For this review, take the finished solid that the model builds, in its own axes (mm). Round coordinates to 2 decimals unless told otherwise and drop trailing zeros. Order: outer loops, then holes, each group sorted by start corner. A loop starts at its lowest first (then second) coordinate and runs counter-clockwise, first axis right, second up.
Autodesk Inventor part; units mm, degrees
ref_plane "YZ Plane" through (0, 0, 0) normal (1, 0, 0) x (0, 1, 0)
ref_plane "XZ Plane" through (0, 0, 0) normal (0, 1, 0) x (-1, 0, 0)
ref_plane "XY Plane" through (0, 0, 0) normal (0, 0, 1) x (1, 0, 0)
sketch "Эскиз1" plane through (0, 0, 0) normal (0, 1, 0) x (-1, 0, 0)
  line L0 (-25, -140.25) -> (25, -140.25)
  line L1 (25, -140.25) -> (25, 140.25)
  line L2 (25, 140.25) -> (-25, 140.25)
  line L3 (-25, 140.25) -> (-25, -140.25)
  line L4 (-25, -140.25) -> (25, 140.25) construction
  line L5 (25, -140.25) -> (-25, 140.25) construction
  circle A0 centre (19.4, 132.25) radius 1.65
  circle A1 centre (19.4, 92.25) radius 1.65
  line L6 (-25, 0) -> (0, 0)
  line L7 (25, 87.25) -> (19.4, 87.25)
  line L8 (19.4, 87.25) -> (19.4, 67.25)
  line L9 (19.4, 67.25) -> (25, 67.25)
  line L10 (25, 67.25) -> (25, 87.25)
  line L11 (-9.2, 133.25) -> (-2.2, 133.25)
  line L12 (-2.2, 133.25) -> (-2.2, 87.25)
  line L13 (-2.2, 87.25) -> (-9.2, 87.25)
  line L14 (-9.2, 87.25) -> (-9.2, 133.25)
  circle A2 centre (19.4, -132.25) radius 1.65
  circle A3 centre (19.4, -92.25) radius 1.65
  line L15 (25, -87.25) -> (19.4, -87.25)
  line L16 (19.4, -87.25) -> (19.4, -67.25)
  line L17 (19.4, -67.25) -> (25, -67.25)
  line L18 (-9.2, -133.25) -> (-2.2, -133.25)
  line L19 (-2.2, -133.25) -> (-2.2, -87.25)
  line L20 (-2.2, -87.25) -> (-9.2, -87.25)
  line L21 (-9.2, -87.25) -> (-9.2, -133.25)
  point P0 (25, -87.25)
  point P1 (25, -67.25)
  dimension "d0" = 50
  dimension "d1" = 280.5
  dimension "d2" = 3.3
  dimension "d3" = 3.3
  dimension "d4" = 5.6
  dimension "d5" = 5.6
  dimension "d6" = 8
  dimension "d7" = 40
  dimension "d8" = 20
  dimension "d9" = 5
  dimension "d10" = 5.6
  dimension "d11" = 7
  dimension "d12" = 46
  dimension "d13" = 7
  dimension "d17" = 28.6
extrude "Выдавливание1" add sketch "Эскиз1" along normal blind 4 contours L3 L2 L1 L7 L8 L9 L17 L16 L15 L0
chamfer "Фаска1" distance 2 angle 45 2 edges at (25, 2, -140.25) (25, 2, 140.25)
chamfer "Фаска2" distance 0.5 angle 45 8 edges at (9.2, 2, 87.25) (2.2, 2, 87.25) (9.2, 2, 133.25) (2.2, 2, 133.25) (2.2, 2, -87.25) (2.2, 2, -133.25) (9.2, 2, -133.25) (9.2, 2, -87.25)
chamfer "Фаска3" distance 1 angle 45 4 edges at (-25, 2, -87.25) (-25, 2, -67.25) (-25, 2, 87.25) (-25, 2, 67.25)
sketch "Эскиз2" plane through (0, 0, 0) normal (0, -1, 0) x (1, 0, 0)
  line L0 (-25, -66.25) -> (-25, 66.25)
  line L1 (-25, -66.25) -> (-34.9, -66.25)
  line L2 (-34.9, -66.25) -> (-34.9, 66.25)
  line L3 (-34.9, 66.25) -> (-25, 66.25)
  line L4 (-25, 66.25) -> (-25, -66.25)
  point P0 (0, 0)
  dimension "d27" = 9.9
extrude "Выдавливание2" add sketch "Эскиз2" against normal blind 4
sketch "Эскиз3" plane through (0, 4, 0) normal (0, 1, 0) x (1, 0, 0)
  line L0 (-34.9, -66.25) -> (-34.9, 66.25)
  line L1 (-34.9, -60.25) -> (-30.9, -60.25)
  line L2 (-30.9, -60.25) -> (-30.9, -48.25)
  line L3 (-30.9, -48.25) -> (-34.9, -48.25)
  line L4 (-34.9, -48.25) -> (-34.9, -60.25)
  line L5 (-34.9, -66.25) -> (-25, -66.25)
  line L6 (-34.9, -42.25) -> (-30.9, -42.25)
  line L7 (-30.9, -42.25) -> (-30.9, -30.25)
  line L8 (-30.9, -30.25) -> (-34.9, -30.25)
  line L9 (-34.9, -30.25) -> (-34.9, -42.25)
  line L10 (-34.9, -24.25) -> (-30.9, -24.25)
  line L11 (-30.9, -24.25) -> (-30.9, -12.25)
  line L12 (-30.9, -12.25) -> (-34.9, -12.25)
  line L13 (-34.9, -12.25) -> (-34.9, -24.25)
  line L14 (-34.9, -6.25) -> (-30.9, -6.25)
  line L15 (-30.9, -6.25) -> (-30.9, 5.75)
  line L16 (-30.9, 5.75) -> (-34.9, 5.75)
  line L17 (-34.9, 5.75) -> (-34.9, -6.25)
  line L18 (-34.9, 11.75) -> (-30.9, 11.75)
  line L19 (-30.9, 11.75) -> (-30.9, 23.75)
  line L20 (-30.9, 23.75) -> (-34.9, 23.75)
  line L21 (-34.9, 23.75) -> (-34.9, 11.75)
  line L22 (-34.9, 29.75) -> (-30.9, 29.75)
  line L23 (-30.9, 29.75) -> (-30.9, 41.75)
  line L24 (-30.9, 41.75) -> (-34.9, 41.75)
  line L25 (-34.9, 41.75) -> (-34.9, 29.75)
  line L26 (-34.9, 47.75) -> (-30.9, 47.75)
  line L27 (-30.9, 47.75) -> (-30.9, 59.75)
  line L28 (-30.9, 59.75) -> (-34.9, 59.75)
  line L29 (-34.9, 59.75) -> (-34.9, 47.75)
  point P0 (0, 0)
  point P1 (-32.9, -60.25)
  point P2 (-32.9, -42.25)
  point P3 (-32.9, -24.25)
  point P4 (-32.9, -6.25)
  point P5 (-32.9, 11.75)
  point P6 (-32.9, 29.75)
  point P7 (-32.9, 47.75)
  dimension "d32" = 4
  dimension "d33" = 12
  dimension "d34" = 6
  dimension "d37" = 18
extrude "Выдавливание3" cut sketch "Эскиз3" against normal blind 4
sketch "Эскиз4" plane through (0, 4, 0) normal (0, 1, 0) x (1, 0, 0)
  circle A0 centre (-4.9309, -102.75) radius 1.6
  circle A1 centre (15.0691, -102.75) radius 1.6
  circle A2 centre (-5.0691, 102.75) radius 1.6
  circle A3 centre (14.9309, 102.75) radius 1.6
  point P0 (0, 0)
extrude "Выдавливание4" cut sketch "Эскиз4" against normal blind 10
sketch "Эскиз5" plane through (0, 4, 0) normal (0, 1, 0) x (1, 0, 0)
  circle A0 centre (21, -58.5) radius 1.6
  circle A1 centre (-11, -58.5) radius 1.6
  circle A2 centre (21, 58.5) radius 1.6
  circle A3 centre (-11, 58.5) radius 1.6
  point P0 (0, 0)
extrude "Выдавливание5" cut sketch "Эскиз5" against normal blind 10
properties part number "фанера_жлектроника_новая"
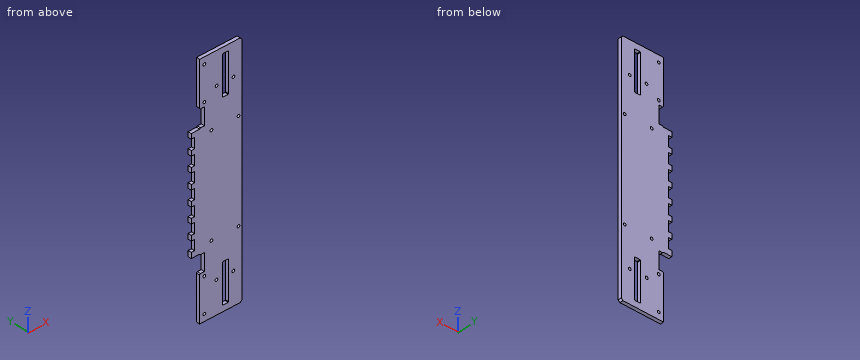
Q1. Take a section at D-D, the plane x = -27.5. State the section outline as (y, z) points.
Q2. Take a section at B-B, the plane z = 83. State the section outline as (x, y) points.
Q3. Take a section at C-C, the plane y = 0.75. Count the separate pieces of the cut face and the enclosed holes in it, plus the area to 3 significant figures.
Q4. Take a section at A-A, the plane z = 123. State the section outline as (x, y) points, plus the area to 3 significant figures.
Q5. Clearance check with flat-ended pins moving along their axes: pin 1 (2 mm diameter, centred on x = -32, y = 2.5, fed in from -Z); pin 2 (2 mm diameter, centred on y = 2.5, z = 51.5, fed in from -X); pin 3 (1.2 mm diameter, centred on y = 2, z = -102, fed in from -X). State where each tip first meets the part, or that it passes through.
Q6. Wall thickness on line 1 (Z direction, x = 21, y = 1.8); line 2 (X direction, y = 1.5, z = 102.75); line 3 (X direction, y = 1.1, z = -132.25): over which ranges is each line inside the solid? List them lowest first.
Working result:
1. outline: (0, -66.25) - (4, -66.25) - (4, 66.25) - (0, 66.25) - close
2. outline: (-19.4, 0) - (25, 0) - (25, 4) - (-19.4, 4) - close
3. separate pieces: 1
3. enclosed holes: 14
3. area: 14,000 mm2
4. outline: (-25, 0) - (2.2, 0) - (2.2, 4) - (-25, 4) - close; (9.2, 0) - (25, 0) - (25, 4) - (9.2, 4) - close
4. area: 172 mm2
5. pin 1: stops at z = -66.25
5. pin 2: stops at x = -30.9
5. pin 3: stops at x = -25
6. line 1: z = -140.25 to -60.1, -56.9 to 56.9, 60.1 to 140.25
6. line 2: x = -25 to -6.53, -3.33 to 2.2, 9.2 to 13.47, 16.67 to 25
6. line 3: x = -25 to -21.05, -17.75 to 2.2, 9.2 to 25
